The listing builds one solid part. Answer for the finished solid, in the listing's coordinates (mm). Coordinates: 2 decimals unless noted, no trailing zeros. Order: outer loops, then holes, each group sorted by start corner. A loop starts at its lowest first (then second) coordinate and runs counter-clockwise, first axis right, second up. Notation, with made-up numbers: (74, 31.25) -> (126, 31.25) arc R29 ccw to (126, 56.25) -> close; hole circle Ø10 at (51.25, 56). An arc over 180 degrees is marked (long way). Answer in a Markdown table with one row per item. Add a question column.
```python
from build123d import *

# Parameters (mm, degrees)
F0_R     = 2
F0_R_2   = 3.05
F1_DEPTH = 2.2
F2_R     = 35
F3_R     = 15
F4_R     = 1.5
F5_R     = 3


with BuildPart() as f1:
    # F0 (on Front) → F1 (new body)
    with BuildSketch(Plane.XZ):
        with BuildLine():
            Line((52.6173001252, 130.7482583531), (41.2109028752, 125.1659909507))
            Line((41.2109028752, 125.1659909507), (20.4584298604, 107.9115033818))
            ThreePointArc((20.4584298604, 107.9115033818), (0, 100.5174507858), (-20.4584298604, 107.9115033818))
            Line((-20.4584298604, 107.9115033818), (-41.2109028752, 125.1659909507))
            Line((-41.2109028752, 125.1659909507), (-52.6173001252, 130.7482583531))
            Line((-52.6173001252, 130.7482583531), (-60.1081627094, 136.9764796956))
            ThreePointArc((-60.1081627094, 136.9764796956), (-70.17561569, 136.6806435954), (-69.4613509604, 126.6342037081))
            Line((-69.4613509604, 126.6342037081), (-65.5419625699, 123.3754577161))
            Line((-65.5419625699, 123.3754577161), (-70.2992250124, 117.6537600959))
            ThreePointArc((-70.2992250124, 117.6537600959), (-70.1188602171, 112.67914718), (-65.1466267703, 112.9162118817))
            Line((-65.1466267703, 112.9162118817), (-61.7026267828, 116.7487230653))
            Line((-61.7026267828, 116.7487230653), (-58.1451833135, 110.6085375713))
            Line((-58.1451833134, 110.6085375713), (-31, 87))
            Line((-31, 87), (31, 87))
            Line((31, 87), (58.1451833134, 110.6085375713))
            Line((58.1451833135, 110.6085375713), (61.7026267828, 116.7487230653))
            Line((61.7026267828, 116.7487230653), (65.1466267703, 112.9162118817))
            ThreePointArc((65.1466267703, 112.9162118817), (70.1188602171, 112.67914718), (70.2992250124, 117.6537600959))
            Line((70.2992250124, 117.6537600959), (65.5419625699, 123.3754577161))
            Line((65.5419625699, 123.3754577161), (69.4613509604, 126.6342037081))
            ThreePointArc((69.4613509604, 126.6342037081), (70.17561569, 136.6806435954), (60.1081627094, 136.9764796956))
            Line((60.1081627094, 136.9764796956), (52.6173001252, 130.7482583531))
        make_face()
        with Locations((-67.7499321664, 115.2556137314)):
            Circle(F0_R, mode=Mode.SUBTRACT)
        with Locations((-65, 132)):
            Circle(F0_R_2, mode=Mode.SUBTRACT)
        with Locations((67.7499321664, 115.2556137314)):
            Circle(F0_R, mode=Mode.SUBTRACT)
        with Locations((65, 132)):
            Circle(F0_R_2, mode=Mode.SUBTRACT)
    extrude(amount=F1_DEPTH)

    # F2
    f2_edges = [f1.edges().sort_by_distance(p)[0] for p in [
        (41.210903, -1.1, 125.165991),
        (-41.210903, -1.1, 125.165991),
    ]]
    fillet(f2_edges, radius=F2_R)

    # F3
    f3_edges = [f1.edges().sort_by_distance(p)[0] for p in [
        (58.145183, -1.1, 110.608538),
        (-58.145183, -1.1, 110.608538),
    ]]
    fillet(f3_edges, radius=F3_R)

    # F4
    f4_edges = [f1.edges().sort_by_distance(p)[0] for p in [
        (-61.702627, -1.1, 116.748723),
        (61.702627, -1.1, 116.748723),
        (-31, -1.1, 87),
    ]]
    fillet(f4_edges, radius=F4_R)

    # F5
    f5_edges = [f1.edges().sort_by_distance(p)[0] for p in [
        (65.541963, -1.1, 123.375458),
        (-65.541963, -1.1, 123.375458),
    ]]
    fillet(f5_edges, radius=F5_R)


solid = f1.part
```
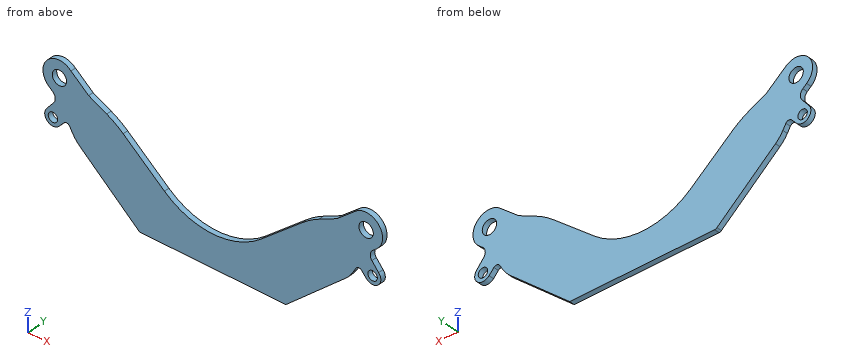
Q1. Given pin 1 (1 mm diameter, centred on y = -0.5, z = 123.5, fed in from +X); pin 2 (10 mm diameter, centred on x = -65, z = 132, fed in from +Y); pin 3 (1 mm diameter, centred on x = -50.5, y = -1, fed in from +Z), each flat-ended and moving along its own axis, determine where each tip first touches the part or whether it passes through.
Q2. A cutting plane is placed at C-C (x = -7.5). Determine the outline of the cut face in (y, z).
Q3. A cutting plane is placed at D-D (x = 23). Determine the outline of the cut face in (y, z).
Q4. Straight lines are drawn through the part: line 1 (X direction, y = -0.95, z = 132); line 2 (X direction, y = -0.6, z = 116); line 3 (Z direction, x = -65, y = -1.7). For each, find the intervals that lie inside material, in ascending order.
Q5. A cutting plane is placed at A-A (z = 132). Determine the outline of the cut face in (x, y), then the cut area to 3 significant figures.
Q6. A cutting plane is placed at B-B (z = 104). Determine the outline of the cut face in (x, y), then the cut area to 3 significant figures.
Returned:
| question | item | result |
|---|---|---|
| 1 | pin 1 | stops at x = 66.94 |
| 1 | pin 2 | stops at y = 0 |
| 1 | pin 3 | stops at z = 129.96 |
| 2 | outline | (-2.2, 87) -> (0, 87) -> (0, 101.41) -> (-2.2, 101.41) -> close |
| 3 | outline | (-2.2, 87) -> (0, 87) -> (0, 110.02) -> (-2.2, 110.02) -> close |
| 4 | line 1 | x = -71.98 to -68.05, -61.95 to -54.12, 54.12 to 61.95, 68.05 to 71.98 |
| 4 | line 2 | x = -71.17 to -69.61, -65.89 to -30.19, 30.19 to 65.89, 69.61 to 71.17 |
| 4 | line 3 | z = 113.08 to 128.95, 135.05 to 138.98 |
| 5 | outline | (-71.98, -2.2) -> (-68.05, -2.2) -> (-68.05, 0) -> (-71.98, 0) -> close; (-61.95, -2.2) -> (-54.12, -2.2) -> (-54.12, 0) -> (-61.95, 0) -> close; (54.12, -2.2) -> (61.95, -2.2) -> (61.95, 0) -> (54.12, 0) -> close; (68.05, -2.2) -> (71.98, -2.2) -> (71.98, 0) -> (68.05, 0) -> close |
| 5 | area | 51.7 mm² |
| 6 | outline | (-50.55, -2.2) -> (-14.52, -2.2) -> (-14.52, 0) -> (-50.55, 0) -> close; (14.52, -2.2) -> (50.55, -2.2) -> (50.55, 0) -> (14.52, 0) -> close |
| 6 | area | 159 mm² |
